Source: CAD feature listing. Evaluate the final solid. Frame: model axes, mm. A direction names the side the tool comes from. Give positions to 0.01 mm unless a question says otherwise; leave off trailing zeros. Order: outer loops, then holes, each group sorted by start corner. A loop starts at its lowest first (then second) coordinate and runs counter-clockwise, first axis right, second up.
```python
from build123d import *

# Parameters (mm, degrees)
SKETCH_1_W          = 10
SKETCH_1_H          = 10
SKETCH_1_W_2        = 8
SKETCH_1_H_2        = 8
EXTRUDE_1_DEPTH     = 210
SKETCH_2_R          = 1.6
CUT_EXTRUDE_1_DEPTH = 211.297408448
SKETCH_3_R          = 1.6
CUT_EXTRUDE_2_DEPTH = 211.297408448
SKETCH_4_R          = 1.6
CUT_EXTRUDE_3_DEPTH = 211.297408448


with BuildPart() as part:
    # ｽｹｯﾁ1 → ﾎﾞｽ - 押し出し1 (new body)
    with BuildSketch(Plane.XY):
        Rectangle(SKETCH_1_W, SKETCH_1_H)
        Rectangle(SKETCH_1_W_2, SKETCH_1_H_2, mode=Mode.SUBTRACT)
    extrude(amount=EXTRUDE_1_DEPTH)

    # ｽｹｯﾁ2 → ｶｯﾄ - 押し出し1 (cut, through all)
    with BuildSketch(Plane.ZY.offset(5)):
        with Locations(Location((5, 0, 0), (0, 0, 270))):
            Circle(SKETCH_2_R)
        with Locations(Location((75, 0, 0), (0, 0, 270))):
            Circle(SKETCH_2_R)
        with Locations(Location((195, 0, 0), (0, 0, 270))):
            Circle(SKETCH_2_R)
    extrude(amount=-CUT_EXTRUDE_1_DEPTH, mode=Mode.SUBTRACT)

    # ｽｹｯﾁ3 → ｶｯﾄ - 押し出し2 (cut, through all)
    with BuildSketch(Plane(origin=(0, 5, 0), x_dir=(1, 0, 0), z_dir=(0, 1, 0))):
        with Locations(Location((0, -15, 0), (0, 0, 270))):
            Circle(SKETCH_3_R)
        with Locations(Location((0, -85, 0), (0, 0, 270))):
            Circle(SKETCH_3_R)
        with Locations(Location((0, -40, 0), (0, 0, 270))):
            Circle(SKETCH_3_R)
    extrude(amount=-CUT_EXTRUDE_2_DEPTH, mode=Mode.SUBTRACT)

    # ｽｹｯﾁ4 → ｶｯﾄ - 押し出し3 (cut, through all)
    with BuildSketch(Plane(origin=(0, 5, 0), x_dir=(1, 0, 0), z_dir=(0, 1, 0))):
        with Locations(Location((0, -205, 0), (0, 0, 270))):
            Circle(SKETCH_4_R)
    extrude(amount=-CUT_EXTRUDE_3_DEPTH, mode=Mode.SUBTRACT)


solid = part.part
```
1) Section query A-A, the plane y = 0. Count the separate pieces of the cut face and the enclosed holes in it, and give its area (3 significant figures).
Report:
separate pieces: 8
enclosed holes: 0
area: 401 mm2
2) Material intervals for L1, parallel to Z at x = -4.35, y = 0; L2, parallel to Y at x = -1, z = 30; L3, parallel to Y at x = 4.5, z = 75, sorted ascending.
Report:
L1: z = 0 to 3.4, 6.6 to 73.4, 76.6 to 193.4, 196.6 to 210
L2: y = -5 to -4, 4 to 5
L3: y = -5 to -1.6, 1.6 to 5
3) Pin query (flat end, axial travel): pin 1 (5 mm diameter, centred on y = 0, z = 75, fed in from -X). Return the tip coordinate at first contact, or that it passes through.
Report:
pin 1: stops at x = -5
4) Section query B-B, the plane z = 59.5. Return the cut outline in (x, y), and give its area (3 significant figures).
Report:
outline: (-5, -5) - (5, -5) - (5, 5) - (-5, 5) - close; hole (-4, -4) - (4, -4) - (4, 4) - (-4, 4) - close
area: 36.0 mm2
5) Reachability of faces 1 (the cylindrical face through (1.08, 4.51, 38.82)), 2 (the flat face through (4, 0, 104)) from +Z, -Z, +X, -X, +Y, -Y: full face, straight path, thin tool, end or side. Return the list, or none.
Report:
face 1: +Y, -Y
face 2: +Z, -Z
6) Draft query along Y for faces 3 (the cylindrical face through (0.07, 4.51, 83.4)), 4 (the flat face through (0, -5, 104)), 5 (the flat face through (0, 5, 104)), 6 (the cylindrical face through (-4.507, 0.208, 76.586)). Return one class per face: +Y half, -Y half, draft (parallel to the pull), parting line (faces both ways), or undercut.
Report:
face 3: draft
face 4: -Y half
face 5: +Y half
face 6: undercut
